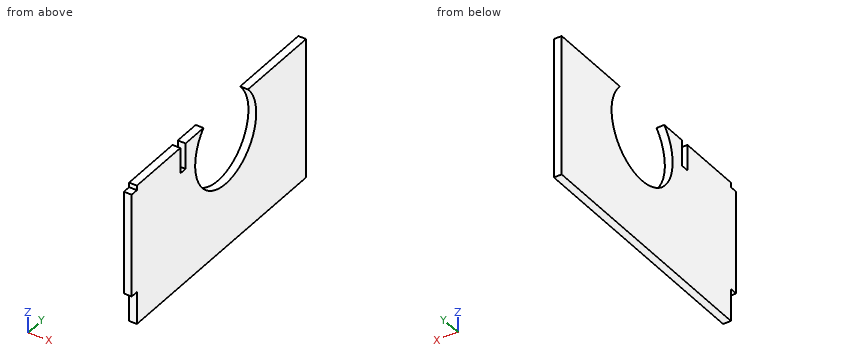
Solid Edge part; units mm, degrees
sketch "Sketch1" plane through (0, 0, 0) normal (1, 0, 0) x (0, 1, 0)
  line L0 (-9.4265, 59.4757) -> (-9.4265, 5.1057)
  line L1 (-9.4265, 5.1057) -> (-106.4265, 5.1057)
  line L2 (-106.4265, 5.1057) -> (-106.4265, 17.6757)
  line L3 (-106.4265, 17.6757) -> (-109.4265, 17.6757)
  line L4 (-109.4265, 17.6757) -> (-109.4265, 57.6757)
  line L5 (-109.4265, 57.6757) -> (-106.4265, 57.6757)
  line L6 (-106.4265, 57.6757) -> (-106.4265, 59.4757)
  line L7 (-106.4265, 59.4757) -> (-81.5265, 59.4757)
  line L8 (-81.5265, 49.4757) -> (-81.5265, 59.4757)
  line L9 (-78.5265, 49.4757) -> (-81.5265, 49.4757)
  line L10 (-78.5265, 59.4757) -> (-78.5265, 49.4757)
  line L11 (-78.5265, 59.4757) -> (-68.2643, 59.4757)
  line L12 (-42.7888, 59.4757) -> (-9.4265, 59.4757)
  arc A0 (-42.7888, 59.4757) -> (-68.2643, 59.4757) centre (-55.5265, 47.4757) cw
  dimension "D1" = 109.4265
  dimension "D2" = 9.4265
  dimension "D3" = 109.4265
  dimension "D4" = 106.4265
  dimension "D5" = 78.5265
  dimension "D6" = 81.5265
extrude "Protrusion1" add sketch "Sketch1" along normal blind 3
properties material "Acier"
Work out the finished part from the listing and answer in its coordinate system (mm). Round coordinates to 2 decimals unless told otherwise and drop trailing zeros. Write each loop counter-clockwise with the first axis right and the second up, starting at its lowest first coordinate (ties: lowest second). Pieces come first, ordered by that corner, then holes. Notation, with made-up numbers: (-27.5, 25) - (23.5, 25) arc R26 ccw to (23.5, 41) - close; hole circle Ø3 at (-18, 33). An arc over 180 degrees is marked (long way). Answer in a Markdown table with one row per item. Add a question column.
1. A cutting plane is placed at A-A, the plane z = 35. Determine the outline of the cut face in (x, y), and give its area (3 significant figures).
2. Find the intervals of material crossed by line 1 along Y through (x, z) = (1.3, 52); line 2 along Y through (x, z) = (0.7, 51); line 3 along Y through (x, z) = (0.6, 48), in increasing order. Write a range as from..to.
3. A cutting plane is placed at B-B, the plane z = 56.5. Determine the outline of the cut face in (x, y).
4. A cutting plane is placed at C-C, the plane y = -39. Determine the outline of the cut face in (x, z), and give its area (3 significant figures).
5. A cutting plane is placed at D-D, the plane x = 1.6. Determine the outline of the cut face in (y, z), and give its area (3 significant figures).
6. Given pin 1 (21 mm diameter, centred on y = -55.53, z = 47.48, fed in from -X); pin 2 (0.9 mm diameter, centred on x = 1.5, y = -107.5, fed in from +Z), each flat-ended and moving along its own axis, determine where each tip first touches the part or whether it passes through.
Worked out:
| question | item | result |
|---|---|---|
| 1 | outline | (0, -109.43) - (3, -109.43) - (3, -67.8) - (0, -67.8) - close; (0, -43.25) - (3, -43.25) - (3, -9.43) - (0, -9.43) - close |
| 1 | area | 226 mm^2 |
| 2 | line 1 | -109.43..-81.53, -78.53..-72.43, -38.62..-9.43 |
| 2 | line 2 | -109.43..-81.53, -78.53..-72.67, -38.39..-9.43 |
| 2 | line 3 | -109.43..-73.02, -38.03..-9.43 |
| 3 | outline | (0, -109.43) - (3, -109.43) - (3, -81.53) - (0, -81.53) - close; (0, -78.53) - (3, -78.53) - (3, -70.52) - (0, -70.52) - close; (0, -40.53) - (3, -40.53) - (3, -9.43) - (0, -9.43) - close |
| 4 | outline | (0, 5.11) - (3, 5.11) - (3, 41.72) - (0, 41.72) - close; (0, 53.23) - (3, 53.23) - (3, 59.48) - (0, 59.48) - close |
| 4 | area | 129 mm^2 |
| 5 | outline | (-109.43, 17.68) - (-106.43, 17.68) - (-106.43, 5.11) - (-9.43, 5.11) - (-9.43, 59.48) - (-42.79, 59.48) arc R17.5 cw (long way) to (-68.26, 59.48) - (-78.53, 59.48) - (-78.53, 49.48) - (-81.53, 49.48) - (-81.53, 59.48) - (-106.43, 59.48) - (-106.43, 57.68) - (-109.43, 57.68) - close |
| 5 | area | 4,500 mm^2 |
| 6 | pin 1 | through |
| 6 | pin 2 | z = 57.68 |
